Could you check a few things on this model? Use its own coordinates, in mm. A direction names the side the tool comes from. Round coordinates to 2 decimals unless told otherwise and drop trailing zeros. Write each loop counter-clockwise with the first axis right and the second up, starting at its lowest first coordinate (ties: lowest second). Pieces come first, ordered by that corner, then holes. Notation, with made-up numbers: (-29.75, 13.25) -> (-1.75, 13.25) arc R10 cw to (-1.75, 25.25) -> close; hole circle Ø3 at (-3, -19). An arc over 180 degrees is marked (long way). Answer in a Markdown table with one row per item.
Solid Edge part; units mm, degrees
sketch "Sketch1" plane through (0, 0, 0) normal (0, -1, 0) x (1, 0, 0)
  line L0 (-27.5, -8) -> (-27.5, 0)
  line L1 (-24, 0) -> (-27.5, 0)
  line L2 (27.5, 0) -> (24, 0)
  line L3 (27.5, 0) -> (27.5, -8)
  line L4 (27.5, -8) -> (37.5, -8)
  line L5 (37.5, -8) -> (37.5, -37.5)
  line L6 (37.5, -37.5) -> (-37.5, -37.5)
  line L7 (-37.5, -37.5) -> (-37.5, -8)
  line L8 (-37.5, -8) -> (-27.5, -8)
  arc A0 (-24, 0) -> (24, 0) centre (0, 0) ccw
extrude "Protrusion1" add sketch "Sketch1" along normal blind 10
sketch "Sketch2" plane through (0, 0, 0) normal (0, -1, 0) x (1, 0, 0)
  line L0 (11.5, -37.5) -> (-11.5, -37.5)
  line L1 (-11.5, -37.5) -> (-8.814, -114.416)
  arc A0 (-8.814, -114.416) -> (-12.3437, -126.4774) centre (-28.8019, -115.114) cw
  arc A1 (8.814, -114.416) -> (12.3437, -126.4774) centre (28.8019, -115.114) ccw
  line L2 (11.5, -37.5) -> (8.814, -114.416)
  arc A2 (-12.3437, -126.4774) -> (12.3437, -126.4774) centre (0, -135) cw
extrude "Protrusão_Extrudada_2" add sketch "Sketch2" along normal blind 8
sketch "Sketch3" plane through (0, 0, 0) normal (0, -1, 0) x (1, 0, 0)
  circle A0 centre (0, -135) radius 9
  circle A1 centre (0, -135) radius 15
extrude "Protrusão_Extrudada_4" add sketch "Sketch3" along normal blind 10
1) For pin 1 (6 mm diameter, centred on x = -4, z = -46, fed in from -Y); pin 2 (2.5 mm diameter, centred on y = -2.5, z = -5.5, fed in from -X); pin 3 (3 mm diameter, centred on x = 18.5, y = -9, fed in from -Z); pin 4 (8 mm diameter, centred on x = -2.5, z = -103.5, fed in from +Y), each with a flat end and sliding along its axis, tell me the tip position at first contact or that it passes through.
Findings:
| item | result |
|---|---|
| pin 1 | stops at y = -8 |
| pin 2 | stops at x = -27.5 |
| pin 3 | stops at z = -37.5 |
| pin 4 | stops at y = 0 |
2) Imagine slicing it at B-B, the plane x = 0. Please give me the cut outline in (y, z).
Findings:
| item | result |
|---|---|
| outline | (-10, -150) -> (0, -150) -> (0, -144) -> (-10, -144) -> close; (-10, -126) -> (0, -126) -> (0, -24) -> (-10, -24) -> (-10, -37.5) -> (-8, -37.5) -> (-8, -120) -> (-10, -120) -> close |
3) Imagine slicing it at C-C, the plane y = -5. Please give me the cut outline in (x, z).
Findings:
| item | result |
|---|---|
| outline | (-37.5, -37.5) -> (-11.5, -37.5) -> (-8.81, -114.42) arc R20 cw to (-12.34, -126.48) arc R15 ccw (long way) to (12.34, -126.48) arc R20 cw to (8.81, -114.42) -> (11.5, -37.5) -> (37.5, -37.5) -> (37.5, -8) -> (27.5, -8) -> (27.5, 0) -> (24, 0) arc R24 cw to (-24, 0) -> (-27.5, 0) -> (-27.5, -8) -> (-37.5, -8) -> close; hole circle Ø18 at (0, -135) |
4) Imagine slicing it at A-A, the plane z = -135. Please give me the cut outline in (x, y).
Findings:
| item | result |
|---|---|
| outline | (-15, -10) -> (-9, -10) -> (-9, 0) -> (-15, 0) -> close; (9, -10) -> (15, -10) -> (15, 0) -> (9, 0) -> close |
5) Imagine slicing it at D-D, the plane z = -18. Please give me the cut outline in (x, y), plus the area to 3 significant figures.
Findings:
| item | result |
|---|---|
| outline | (-37.5, -10) -> (-15.87, -10) -> (-15.87, 0) -> (-37.5, 0) -> close; (15.87, -10) -> (37.5, -10) -> (37.5, 0) -> (15.87, 0) -> close |
| area | 433 mm^2 |
6) Thinking about a two-plate mould opening in X: for faces 4 (the face through (-26, -5, 0)), 5 (the face through (-1.172, -4.93, -143.923)), 6 (the face through (37.5, -5, -23)), 7 (the face through (-27.5, -5, -4)), which applies, +X half, -X half, draft (parallel to the pull), parting line (faces both ways), or undercut?
Findings:
| item | result |
|---|---|
| face 4 | draft |
| face 5 | undercut |
| face 6 | +X half |
| face 7 | -X half |
7) For faces 1 (the face through (-9.582, -3.944, -120.645)), 2 (the face through (-33, -5, -8)), 3 (the face through (32, -5, -8)), which set-ups out of +Z, -Z, +X, -X, +Y, -Y let a thin tool reach every point of the face, with its end or its side?
Findings:
| item | result |
|---|---|
| face 1 | -X, +Y, -Y |
| face 2 | +Z, -X, +Y, -Y |
| face 3 | +Z, +X, +Y, -Y |
8) Please list where these lines run through material, in increasing order: line 1 (Z direction, x = 0, y = -2.5); line 2 (X direction, y = -8.25, z = -135.5); line 3 (Z direction, x = 4, y = -9).
Findings:
| item | result |
|---|---|
| line 1 | z = -150 to -144, -126 to -24 |
| line 2 | x = -14.99 to -8.99, 8.99 to 14.99 |
| line 3 | z = -149.46 to -143.06, -126.94 to -120.54, -37.5 to -23.66 |
